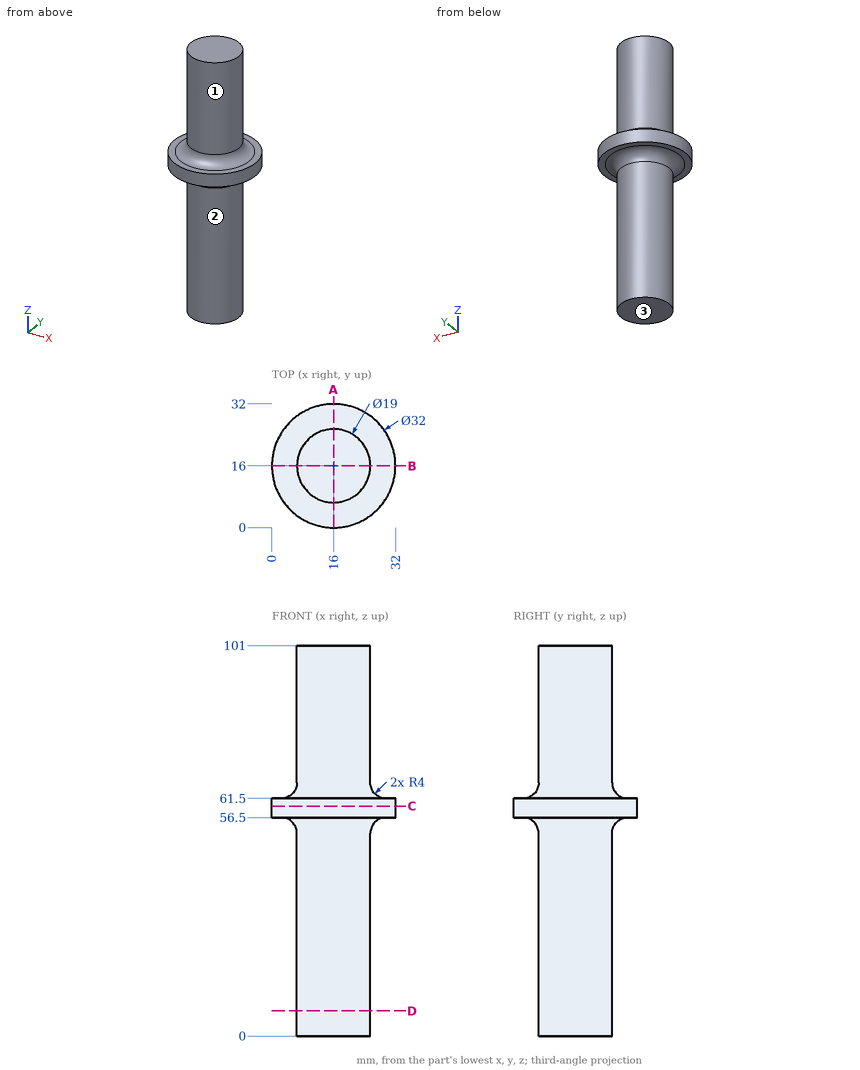
The drawing under review shows one solid part. Ordinate dimensions are in mm from its lowest x, y, z. A direction names the side the tool comes from. Round coordinates to 2 decimals unless told otherwise and drop trailing zeros. Loops run counter-clockwise (first coordinate to the right, second up) from the corner with the lowest first, then second, coordinate; pieces in that order, holes last. Notation, with made-up numbers: (-29.75, 42) -> (18.25, 42) arc R8 cw to (18.25, 55) -> close; hole circle Ø8 at (-22.5, -17.75). An arc over 180 degrees is marked (long way). One line per question, with ' | ' between items. Start each with the question number.
Item 1: Wall thickness on line 1 along Z through (x, y) = (30, 11.5); line 2 along X through (y, z) = (10.5, 58.5); line 3 along X through (y, z) = (15, 53.5): over which ranges is each line inside the solid? List them lowest first. Write a range as [from, to].
Item 2: Add section C-C, the plane z = 59.5. Write out the cut boundary in (x, y).
Item 3: For pin 1 (6 mm diameter, centred on y = 22, z = 20.5, fed in from +X); pin 2 (2 mm diameter, centred on x = 11, z = 13, fed in from -Y); pin 3 (1 mm diameter, centred on x = 7.5, y = 11.5, fed in from -Z); pin 4 (1 mm diameter, centred on y = 8, z = 65, fed in from +X), all flat-tipped, find the tip position at first contact; note any pin that passes through.
Item 4: Add section A-A, the plane x = 16. Write out the cut boundary in (y, z).
Item 5: Add section D-D, the plane z = 6.5. Write out the cut boundary in (x, y).
Item 6: Machinability: for the marked faces 1, 2 and 3, which of the approach directions +Z, -Z, +X, -X, +Y, -Y give a long, thin tool a straight path to every point of the face, cutting with its end or side? Answer none if there is none.
Return value:
1) line 1: z = [56.5, 61.5] | line 2: x = [0.98, 31.02] | line 3: x = [6.43, 25.57]
2) outline: circle Ø32 at (16, 16)
3) pin 1: stops at x = 25.01 | pin 2: stops at y = 7.38 | pin 3: stops at z = 0 | pin 4: stops at x = 21.89
4) outline: (0, 56.5) -> (2.5, 56.5) arc R4 cw to (6.5, 52.5) -> (6.5, 0) -> (25.5, 0) -> (25.5, 52.5) arc R4 cw to (29.5, 56.5) -> (32, 56.5) -> (32, 61.5) -> (29.5, 61.5) arc R4 cw to (25.5, 65.5) -> (25.5, 101) -> (6.5, 101) -> (6.5, 65.5) arc R4 cw to (2.5, 61.5) -> (0, 61.5) -> close
5) outline: circle Ø19 at (16, 16)
6) face 1: +Z | face 2: -Z | face 3: -Z, +X, -X, +Y, -Y
